Autodesk Inventor part; units mm, degrees
ref_plane "YZ Plane" through (0, 0, 0) normal (1, 0, 0) x (0, 1, 0)
ref_plane "XZ Plane" through (0, 0, 0) normal (0, 1, 0) x (-1, 0, 0)
ref_plane "XY Plane" through (0, 0, 0) normal (0, 0, 1) x (1, 0, 0)
sketch "Sketch5" plane through (0, 0, 0) normal (0, 0, 1) x (1, 0, 0)
  line L0 (-20, -20) -> (20, -20)
  line L1 (20, -20) -> (20, 20)
  line L2 (20, 20) -> (-20, 20)
  line L3 (-20, 20) -> (-20, -20)
  line L4 (-20, -20) -> (20, 20) construction
  line L5 (20, -20) -> (-20, 20) construction
  point P0 (0, 0)
  dimension "d13" = 40
  dimension "d14" = 40
extrude "Extrusion5" add sketch "Sketch5" against normal blind 50
sketch "Sketch6" plane through (0, 0, 0) normal (0, 0, 1) x (1, 0, 0)
  circle A0 centre (0, 0) radius 10.05
  dimension "d17" = 20.1
extrude "Extrusion6" cut sketch "Sketch6" against normal blind 40
sketch "Sketch9" plane through (0, 0, -50) normal (0, 0, -1) x (-1, 0, 0)
  line L0 (-10.05, 10.05) -> (10.05, 10.05)
  line L1 (10.05, 10.05) -> (10.05, -10.05)
  line L2 (10.05, -10.05) -> (-10.05, -10.05)
  line L3 (-10.05, -10.05) -> (-10.05, 10.05)
  line L4 (-10.05, 10.05) -> (10.05, -10.05) construction
  line L5 (10.05, 10.05) -> (-10.05, -10.05) construction
  point P0 (0, 0)
  dimension "d28" = 20.1
  dimension "d29" = 20.1
extrude "Extrusion9" cut sketch "Sketch9" against normal blind 5
sketch "Sketch10" plane through (20, -20, 0) normal (1, 0, 0) x (0, 0, -1)
  line L0 (40, 0) -> (50, 0)
  line L1 (50, 0) -> (50, 40)
  line L2 (50, 40) -> (40, 40)
  line L3 (40, 40) -> (40, 0)
  line L4 (40, 0) -> (50, 40) construction
  line L5 (50, 0) -> (40, 40) construction
  line L6 (50, 40) -> (50, 0)
  line L7 (0, 40) -> (50, 40)
  line L8 (0, 0) -> (50, 0)
  point P0 (0, 20)
  point P1 (45, 20)
  dimension "d32" = 10
extrude "Extrusion10" add sketch "Sketch10" along normal blind 15
mirror "Mirror2" about plane through (0, 0, 0) normal (1, 0, 0) of "Extrusion10"
sketch "Sketch11" plane through (0, 0, -50) normal (0, 0, -1) x (-1, 0, 0)
  circle A0 centre (-27.5, 10) radius 2.05
  line L0 (-35, 20) -> (35, 20)
  line L1 (-35, -20) -> (-35, 20)
  circle A1 centre (-27.5, -10) radius 2.05
  circle A2 centre (27.5, -10) radius 2.05
  circle A3 centre (27.5, 10) radius 2.05
  line L2 (35, -20) -> (-35, -20)
  line L3 (35, -20) -> (35, 20)
  point P0 (0, 0)
  dimension "d35" = 4.1
  dimension "d36" = 10
  dimension "d37" = 7.5
  dimension "d38" = 4.1
  dimension "d39" = 4.1
  dimension "d41" = 4.1
  dimension "d42" = 10
  dimension "d43" = 7.5
  dimension "d44" = 7.5
  dimension "d45" = 7.5
  dimension "d46" = 10
  dimension "d47" = 10
extrude "Extrusion11" cut sketch "Sketch11" against normal through all contours A0 | A1 | A2 | A3
sketch "Sketch12" plane through (20, -20, -40) normal (0, 0, 1) x (1, 0, 0)
  circle A0 centre (7.5, 30) radius 2.05
  circle A1 centre (7.5, 10) radius 2.05
  circle A2 centre (-47.5, 10) radius 2.05
  circle A3 centre (-47.5, 30) radius 2.05
  circle A4 centre (7.5, 30) radius 5
  circle A5 centre (7.5, 10) radius 5
  circle A6 centre (-47.5, 30) radius 5
  circle A7 centre (-47.5, 10) radius 5
  point P0 (-20, 20)
  dimension "d50" = 10
  dimension "d51" = 10
  dimension "d52" = 10
  dimension "d53" = 10
extrude "Extrusion12" cut sketch "Sketch12" against normal blind 5
sketch "Sketch13" plane through (20, -20, 0) normal (1, 0, 0) x (0, 0, -1)
  circle A0 centre (30, 20) radius 3.1
  line L0 (40, 40) -> (40, 0)
  point P0 (0, 20)
  point P1 (40, 20)
  dimension "d56" = 6.2
  dimension "d57" = 10
extrude "Extrusion13" cut sketch "Sketch13" against normal through all
sketch "Sketch14" plane through (20, -20, 0) normal (1, 0, 0) x (0, 0, -1)
  line L0 (37.5, 27.5) -> (22.5, 27.5)
  line L1 (22.5, 27.5) -> (22.5, 12.5)
  line L2 (22.5, 12.5) -> (37.5, 12.5)
  line L3 (37.5, 12.5) -> (37.5, 27.5)
  line L4 (37.5, 27.5) -> (22.5, 12.5) construction
  line L5 (22.5, 27.5) -> (37.5, 12.5) construction
  line L6 (40, 0) -> (40, 40)
  circle A0 centre (30, 20) radius 3.1
  point P0 (0, 20)
  dimension "d60" = 15
  dimension "d61" = 15
extrude "Extrusion14" cut sketch "Sketch14" against normal blind 5 contours L3 L2 L1 L0 | A0
mirror "Mirror3" about plane through (0, 0, 0) normal (1, 0, 0) of "Extrusion14"
sketch "Sketch15" plane through (0, 0, 0) normal (0, 0, 1) x (1, 0, 0)
  line L0 (-20, -20) -> (20, -20)
  line L1 (20, -20) -> (20, 20)
  line L2 (20, 20) -> (-20, 20)
  line L3 (-20, 20) -> (-20, -20)
  line L4 (-20, -20) -> (20, 20) construction
  line L5 (20, -20) -> (-20, 20) construction
  circle A0 centre (0, 0) radius 10.05
  circle A1 centre (0, 0) radius 10.05
  line L6 (20, 20) -> (-20, 20)
  line L7 (-20, 20) -> (-20, -20)
  line L8 (-20, -20) -> (20, -20)
  line L9 (20, -20) -> (20, 20)
extrude "Extrusion15" cut sketch "Sketch15" against normal blind 18
properties part number "linear_bracket" material "ABS Plastic"
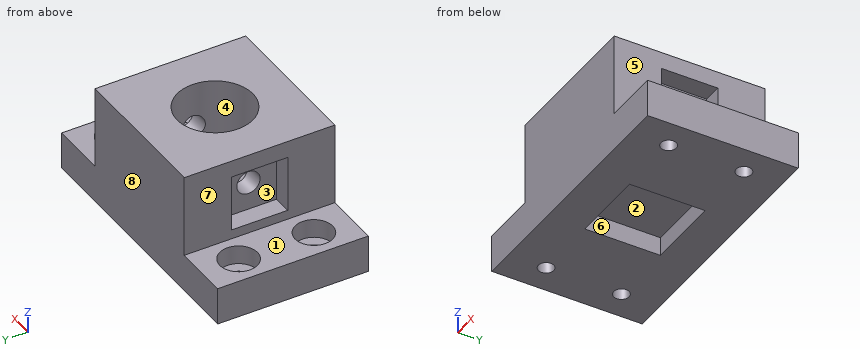
Input: part model. Units: mm. Frame: model coordinates. Face numbers are marked on the shaded views. A direction names the side the tool comes from. Give positions to 0.01 mm unless a question says otherwise; leave off trailing zeros. Write each loop counter-clockwise with the first axis right and the second up, starting at its lowest first coordinate (ties: lowest second). Pieces come first, ordered by that corner, then holes. Notation, with made-up numbers: (65.5, -16.75) - (79.5, -16.75) arc R17 cw to (79.5, 3.25) - close; hole circle Ø3 at (-3, -29.5). An arc over 180 degrees is marked (long way). Write item = value, one per line. Start each with the question number.
1. Mould query, pull axis Y, two halves, no side actions, for the marked faces 6, 7 and 8. Classes: released by +Y, released by -Y, zero draft, split by the parting line, or undercut.
2. Ray query, L1, parallel to Y at x = -27.5, z = -42.6; L2, parallel to Y at x = -27.5, z = -46.45; L3, parallel to Y at x = -11.75, z = -30. Return the intervals inside material, ascending.
3. Access query for the marked faces 1, 2, 3, 4 and 5. Directions: +Z, -Z, +X, -X, +Y, -Y. A direction counts if a zero-diameter tool reaches every point of the face in a straight line with its end or side. Return the directions, or none.
4. Section query B-B, the plane y = 0. Count the separate pieces of the cut face and the enclosed holes in it, then the cut area to 3 significant figures.
5. Section query A-A, the plane z = -30. Output: boundary loops of the cut face in (x, y), then the cut area to 3 significant figures.
6. Section query C-C, the plane x = -16. Output: boundary loops of the cut face in (y, z).
7. Section query D-D, the plane z = -25. Output: boundary loops of the cut face in (x, y).
8. First-contact query: pin 1 Ø11 at (y, z) = (-2.5, -32.5) entering from +X; pin 2 Ø6 at (x, y) = (-27.5, 10) entering from +Z; pin 3 Ø16.5 at (x, y) = (-30.5, -7) entering from +Z; pin 4 Ø5 at (y, z) = (13, -38) entering from -X. Flat tips, straight axial feed; report the tip coordinate or a pass-through.
Check sheet entries:
q1.face_6 = undercut
q1.face_7 = zero draft
q1.face_8 = released by +Y
q2.L1 = -20 to -15, -5 to 5, 15 to 20
q2.L2 = -20 to -12.05, -7.95 to 7.95, 12.05 to 20
q2.L3 = -20 to -3.1, 3.1 to 20
q3.face_1 = +Z, -X, +Y, -Y
q3.face_2 = -Z
q3.face_3 = -X
q3.face_4 = +Z
q3.face_5 = +Z, +X, +Y, -Y
q4.separate_pieces = 3
q4.enclosed_holes = 0
q4.area = 826 mm2
q5.outline = (-20, -20) - (20, -20) - (20, -7.5) - (15, -7.5) - (15, -3.1) - (9.56, -3.1) arc R10.05 cw to (-9.56, -3.1) - (-15, -3.1) - (-15, -7.5) - (-20, -7.5) - close; (-20, 7.5) - (-15, 7.5) - (-15, 3.1) - (-9.56, 3.1) arc R10.05 cw to (9.56, 3.1) - (15, 3.1) - (15, 7.5) - (20, 7.5) - (20, 20) - (-20, 20) - close
q5.area = 1,070 mm2
q6.outline = (-20, -50) - (20, -50) - (20, -18) - (-20, -18) - close; hole (-7.5, -37.5) - (7.5, -37.5) - (7.5, -22.5) - (-7.5, -22.5) - close
q7.outline = (-20, -20) - (20, -20) - (20, -7.5) - (15, -7.5) - (15, 7.5) - (20, 7.5) - (20, 20) - (-20, 20) - (-20, 7.5) - (-15, 7.5) - (-15, -7.5) - (-20, -7.5) - close; hole circle Ø20.1 at (0, 0)
q8.pin_1 = 20
q8.pin_2 = -45
q8.pin_3 = -40
q8.pin_4 = -35
